CAD build for the part. Positions are in the model's coordinates, mm. A direction names the side the tool comes from. Give positions to 0.01 mm unless a question says otherwise; leave off trailing zeros. Order: outer loops, then holes, each group sorted by start corner. A loop starts at its lowest first (then second) coordinate and runs counter-clockwise, first axis right, second up. Notation, with made-up numbers: (45.25, 51) -> (80.25, 51) arc R14 ccw to (80.25, 70) -> close; hole circle Ø9 at (64.25, -19.75). An arc over 180 degrees is marked (long way). Answer as CSV lines item,"result".
```python
from build123d import *

# Parameters (mm, degrees)
SKETCH1_R           = 1.6
BOSS_EXTRUDE1_DEPTH = 3.5
SKETCH2_W           = 143
SKETCH2_H           = 73
BOSS_EXTRUDE2_DEPTH = 60
CUT_EXTRUDE1_DEPTH  = 127.71720483
CUT_EXTRUDE2_REACH  = 169.727
SKETCH5_W           = 15
SKETCH5_H           = 13.306266554
SKETCH6_R           = 2.25
CUT_EXTRUDE3_DEPTH  = 20


with BuildPart() as part:
    # Sketch1 → Boss-Extrude1 (new body)
    with BuildSketch(Plane(origin=(0, 0, 0), x_dir=(1, 0, 0), z_dir=(0, 1, 0))):
        with BuildLine():
            Line((-73, -40), (73, -40))
            ThreePointArc((73, -40), (74.414213562, -39.414213562), (75, -38))
            Line((75, -38), (75, 38))
            ThreePointArc((75, 38), (74.414213562, 39.414213562), (73, 40))
            Line((73, 40), (-73, 40))
            ThreePointArc((-73, 40), (-74.414213562, 39.414213562), (-75, 38))
            Line((-75, 38), (-75, -38))
            ThreePointArc((-75, -38), (-74.414213562, -39.414213562), (-73, -40))
        make_face()
        with Locations(Location((-25, 26.605, 0), (0, 0, 270))):
            Circle(SKETCH1_R, mode=Mode.SUBTRACT)
        with Locations(Location((49.93, 26.605, 0), (0, 0, 270))):
            Circle(SKETCH1_R, mode=Mode.SUBTRACT)
        with Locations(Location((49.93, -26.605, 0), (0, 0, 270))):
            Circle(SKETCH1_R, mode=Mode.SUBTRACT)
        with Locations(Location((-25, -26.605, 0), (0, 0, 270))):
            Circle(SKETCH1_R, mode=Mode.SUBTRACT)
        with Locations(Location((-45, 0, 0), (0, 0, 270))):
            Circle(SKETCH1_R, mode=Mode.SUBTRACT)
        with Locations(Location((35, 0, 0), (0, 0, 270))):
            Circle(SKETCH1_R, mode=Mode.SUBTRACT)
    extrude(amount=BOSS_EXTRUDE1_DEPTH)

    # Sketch2 → Boss-Extrude2 (add)
    # profile 1 of 5: a face of its own
    with BuildSketch(Plane(origin=(0, 3.5, 0), x_dir=(1, 0, 0), z_dir=(0, 1, 0))):
        with BuildLine():
            Line((73, 40), (-73, 40))
            ThreePointArc((-73, 40), (-74.414213562, 39.414213562), (-75, 38))
            Line((-75, 38), (-75, -38))
            ThreePointArc((-75, -38), (-74.414213562, -39.414213562), (-73, -40))
            Line((-73, -40), (73, -40))
            ThreePointArc((73, -40), (74.414213562, -39.414213562), (75, -38))
            Line((75, -38), (75, 38))
            ThreePointArc((75, 38), (74.414213562, 39.414213562), (73, 40))
        make_face()
        Rectangle(SKETCH2_W, SKETCH2_H, mode=Mode.SUBTRACT)
    # profile 2 of 5: a face of its own
    with BuildSketch(Plane(origin=(0, 3.5, 0), x_dir=(1, 0, 0), z_dir=(0, 1, 0))):
        with BuildLine():
            Line((-67.5, 36.5), (-71.5, 36.5))
            Line((-71.5, 36.5), (-71.5, 32.5))
            ThreePointArc((-71.5, 32.5), (-68.671572875, 33.671572875), (-67.5, 36.5))
        make_face()
    # profile 3 of 5: a face of its own
    with BuildSketch(Plane(origin=(0, 3.5, 0), x_dir=(1, 0, 0), z_dir=(0, 1, 0))):
        with BuildLine():
            ThreePointArc((-67.5, -36.5), (-68.671572875, -33.671572875), (-71.5, -32.5))
            Line((-71.5, -32.5), (-71.5, -36.5))
            Line((-71.5, -36.5), (-67.5, -36.5))
        make_face()
    # profile 4 of 5: a face of its own
    with BuildSketch(Plane(origin=(0, 3.5, 0), x_dir=(1, 0, 0), z_dir=(0, 1, 0))):
        with BuildLine():
            Line((71.5, 36.5), (67.5, 36.5))
            ThreePointArc((67.5, 36.5), (68.671572875, 33.671572875), (71.5, 32.5))
            Line((71.5, 32.5), (71.5, 36.5))
        make_face()
    # profile 5 of 5: a face of its own
    with BuildSketch(Plane(origin=(0, 3.5, 0), x_dir=(1, 0, 0), z_dir=(0, 1, 0))):
        with BuildLine():
            ThreePointArc((71.5, -32.5), (68.671572875, -33.671572875), (67.5, -36.5))
            Line((67.5, -36.5), (71.5, -36.5))
            Line((71.5, -36.5), (71.5, -32.5))
        make_face()
    extrude(amount=BOSS_EXTRUDE2_DEPTH)

    # Sketch3 → Cut-Extrude1 (cut, through all)
    with BuildSketch(Plane.XY.offset(40)):
        with BuildLine():
            Line((63.32083214, 17.25), (63.32083214, 53.25))
            ThreePointArc((63.32083214, 53.25), (60, 56.57083214), (56.67916786, 53.25))
            Line((56.67916786, 53.25), (56.67916786, 17.25))
            ThreePointArc((56.67916786, 17.25), (60, 13.92916786), (63.32083214, 17.25))
        make_face()
        with BuildLine():
            Line((48.32083214, 17.25), (48.32083214, 53.25))
            ThreePointArc((48.32083214, 53.25), (45, 56.57083214), (41.67916786, 53.25))
            Line((41.67916786, 53.25), (41.67916786, 17.25))
            ThreePointArc((41.67916786, 17.25), (45, 13.92916786), (48.32083214, 17.25))
        make_face()
        with BuildLine():
            Line((33.32083214, 17.25), (33.32083214, 53.25))
            ThreePointArc((33.32083214, 53.25), (30, 56.57083214), (26.67916786, 53.25))
            Line((26.67916786, 53.25), (26.67916786, 17.25))
            ThreePointArc((26.67916786, 17.25), (30, 13.92916786), (33.32083214, 17.25))
        make_face()
        with BuildLine():
            Line((18.32083214, 17.25), (18.32083214, 53.25))
            ThreePointArc((18.32083214, 53.25), (15, 56.57083214), (11.67916786, 53.25))
            Line((11.67916786, 53.25), (11.67916786, 17.25))
            ThreePointArc((11.67916786, 17.25), (15, 13.92916786), (18.32083214, 17.25))
        make_face()
        with BuildLine():
            Line((3.32083214, 17.25), (3.32083214, 53.25))
            ThreePointArc((3.32083214, 53.25), (0, 56.57083214), (-3.32083214, 53.25))
            Line((-3.32083214, 53.25), (-3.32083214, 17.25))
            ThreePointArc((-3.32083214, 17.25), (0, 13.92916786), (3.32083214, 17.25))
        make_face()
        with BuildLine():
            Line((-11.67916786, 17.25), (-11.67916786, 53.25))
            ThreePointArc((-11.67916786, 53.25), (-15, 56.57083214), (-18.32083214, 53.25))
            Line((-18.32083214, 53.25), (-18.32083214, 17.25))
            ThreePointArc((-18.32083214, 17.25), (-15, 13.92916786), (-11.67916786, 17.25))
        make_face()
        with BuildLine():
            Line((-26.67916786, 17.25), (-26.67916786, 53.25))
            ThreePointArc((-26.67916786, 53.25), (-30, 56.57083214), (-33.32083214, 53.25))
            Line((-33.32083214, 53.25), (-33.32083214, 17.25))
            ThreePointArc((-33.32083214, 17.25), (-30, 13.92916786), (-26.67916786, 17.25))
        make_face()
        with BuildLine():
            Line((-41.67916786, 17.25), (-41.67916786, 53.25))
            ThreePointArc((-41.67916786, 53.25), (-45, 56.57083214), (-48.32083214, 53.25))
            Line((-48.32083214, 53.25), (-48.32083214, 17.25))
            ThreePointArc((-48.32083214, 17.25), (-45, 13.92916786), (-41.67916786, 17.25))
        make_face()
        with BuildLine():
            Line((-56.67916786, 17.25), (-56.67916786, 53.25))
            ThreePointArc((-56.67916786, 53.25), (-60, 56.57083214), (-63.32083214, 53.25))
            Line((-63.32083214, 53.25), (-63.32083214, 17.25))
            ThreePointArc((-63.32083214, 17.25), (-60, 13.92916786), (-56.67916786, 17.25))
        make_face()
    extrude(amount=-CUT_EXTRUDE1_DEPTH, mode=Mode.SUBTRACT)

    # Sketch5 → Cut-Extrude2 (cut, up to next)
    with BuildSketch(Plane.ZY.offset(75), mode=Mode.PRIVATE) as cut_extrude2_sk1:
        with Locations((-16.5, 22.153133277)):
            Rectangle(SKETCH5_W, SKETCH5_H)
    cut_extrude2_tool1 = extrude(cut_extrude2_sk1.sketch, amount=-CUT_EXTRUDE2_REACH, mode=Mode.PRIVATE) & part.part
    # Sketch5 → Cut-Extrude2 (cut, up to next)
    with BuildSketch(Plane.ZY.offset(75), mode=Mode.PRIVATE) as cut_extrude2_sk2:
        with BuildLine():
            Line((30, 35), (-30, 35))
            ThreePointArc((-30, 35), (-32.5, 32.5), (-30, 30))
            Line((-30, 30), (30, 30))
            ThreePointArc((30, 30), (32.5, 32.5), (30, 35))
        make_face()
    cut_extrude2_tool2 = extrude(cut_extrude2_sk2.sketch, amount=-CUT_EXTRUDE2_REACH, mode=Mode.PRIVATE) & part.part
    add(cut_extrude2_tool1.solids().sort_by_distance((-75, 22.153133, -16.5))[0], mode=Mode.SUBTRACT)
    add(cut_extrude2_tool2.solids().sort_by_distance((-75, 32.5, 0))[0], mode=Mode.SUBTRACT)

    # Sketch6 → Cut-Extrude3 (cut)
    with BuildSketch(Plane(origin=(0, 63.5, 0), x_dir=(1, 0, 0), z_dir=(0, 1, 0))):
        with Locations(Location((-71.542893219, 36.542893219, 0), (0, 0, 270))):
            Circle(SKETCH6_R)
        with Locations(Location((71.542893219, 36.542893219, 0), (0, 0, 90))):
            Circle(SKETCH6_R)
        with Locations(Location((71.542893219, -36.542893219, 0), (0, 0, 270))):
            Circle(SKETCH6_R)
        with Locations(Location((-71.542893219, -36.542893219, 0), (0, 0, 90))):
            Circle(SKETCH6_R)
    extrude(amount=-CUT_EXTRUDE3_DEPTH, mode=Mode.SUBTRACT)


solid = part.part
```
1) Wall check: line 1 along X through (y, z) = (2, 0); line 2 along Z through (x, y) = (64, 12.5); line 3 along X through (y, z) = (20, 18). Give the ranges that are in metal, low to high. Write a range as [from, to].
Data:
line 1,"x = [-75, -46.6], [-43.4, 33.4], [36.6, 75]"
line 2,"z = [-40, -36.5], [36.5, 40]"
line 3,"x = [-75, -71.5], [71.5, 75]"
2) Which spindle directions (+Z, -Z, +X, -X, +Y, -Y) get a long thin tool onto all of the face, cutting with end or side? Do faces 3 (the flat face through (-73, 28.806, -17)), 4 (the cylindrical face through (68.641, 33.08, -33.703)), 5 (the flat face through (17, 10, -40)), 6 (the flat face through (-3.321, 36, 38)). Say none if no direction does.
Data:
face 3,"-X"
face 4,"+Y"
face 5,"-Z, +X, -X, +Y, -Y"
face 6,"+Z, -Z"
3) Band-saw the part on C-C, the plane z = -15. Write the cut outline in (x, y), then the cut area to 3 significant figures.
Data:
outline,"(-75, 0) -> (75, 0) -> (75, 63.5) -> (71.5, 63.5) -> (71.5, 3.5) -> (-71.5, 3.5) -> (-71.5, 15.5) -> (-75, 15.5) -> close; (-75, 28.81) -> (-71.5, 28.81) -> (-71.5, 30) -> (-75, 30) -> close; (-75, 35) -> (-71.5, 35) -> (-71.5, 63.5) -> (-75, 63.5) -> close"
area,"881 mm2"
4) Pull direction X, two halves, no side cores. Call faces 1 (the cylindrical face through (-14.93, 56.57, -38.23)), 2 (the flat face through (-73, 15.5, -17)): pulls with the +X half, pulls with the -X half, needs draft (parallel to the pull), parting line crosses it, or undercut.
Data:
face 1,"undercut"
face 2,"needs draft"
5) Band-saw the part on D-D, the plane x = -60. Write the cut outline in (y, z), then the cut area to 3 significant figures.
Data:
outline,"(0, -40) -> (13.93, -40) -> (13.93, -36.5) -> (3.5, -36.5) -> (3.5, 36.5) -> (13.93, 36.5) -> (13.93, 40) -> (0, 40) -> close; (56.57, -40) -> (63.5, -40) -> (63.5, -36.5) -> (56.57, -36.5) -> close; (56.57, 36.5) -> (63.5, 36.5) -> (63.5, 40) -> (56.57, 40) -> close"
area,"402 mm2"
6) Band-saw the part on A-A, the plane z = 0. Write the cut outline in (x, y).
Data:
outline,"(-75, 0) -> (-46.6, 0) -> (-46.6, 3.5) -> (-71.5, 3.5) -> (-71.5, 30) -> (-75, 30) -> close; (-75, 35) -> (-71.5, 35) -> (-71.5, 63.5) -> (-75, 63.5) -> close; (-43.4, 0) -> (33.4, 0) -> (33.4, 3.5) -> (-43.4, 3.5) -> close; (36.6, 0) -> (75, 0) -> (75, 63.5) -> (71.5, 63.5) -> (71.5, 3.5) -> (36.6, 3.5) -> close"
7) Pin check, flat tips, straight feed: P1, Ø4, axis at x = 71.54, z = 36.54, coming from the +Y side; P2, Ø1, axis at x = 3, z = -5.5, coming from the +Y side; P3, Ø1.8, axis at y = 32.5, z = -39, coming from the +X side; P4, Ø2.5, axis at x = 49.93, z = -26.605, coming from the +Y side. Stop position of each tip, or through.
Data:
P1,"stops at y = 43.5"
P2,"stops at y = 3.5"
P3,"stops at x = 75"
P4,"passes through"
8) Band-saw the part on B-B, the plane x = -45. Write the cut outline in (y, z), then the cut area to 3 significant figures.
Data:
outline,"(0, -40) -> (13.93, -40) -> (13.93, -36.5) -> (3.5, -36.5) -> (3.5, -1.6) -> (0, -1.6) -> close; (0, 1.6) -> (3.5, 1.6) -> (3.5, 36.5) -> (13.93, 36.5) -> (13.93, 40) -> (0, 40) -> close; (56.57, -40) -> (63.5, -40) -> (63.5, -36.5) -> (56.57, -36.5) -> close; (56.57, 36.5) -> (63.5, 36.5) -> (63.5, 40) -> (56.57, 40) -> close"
area,"390 mm2"
